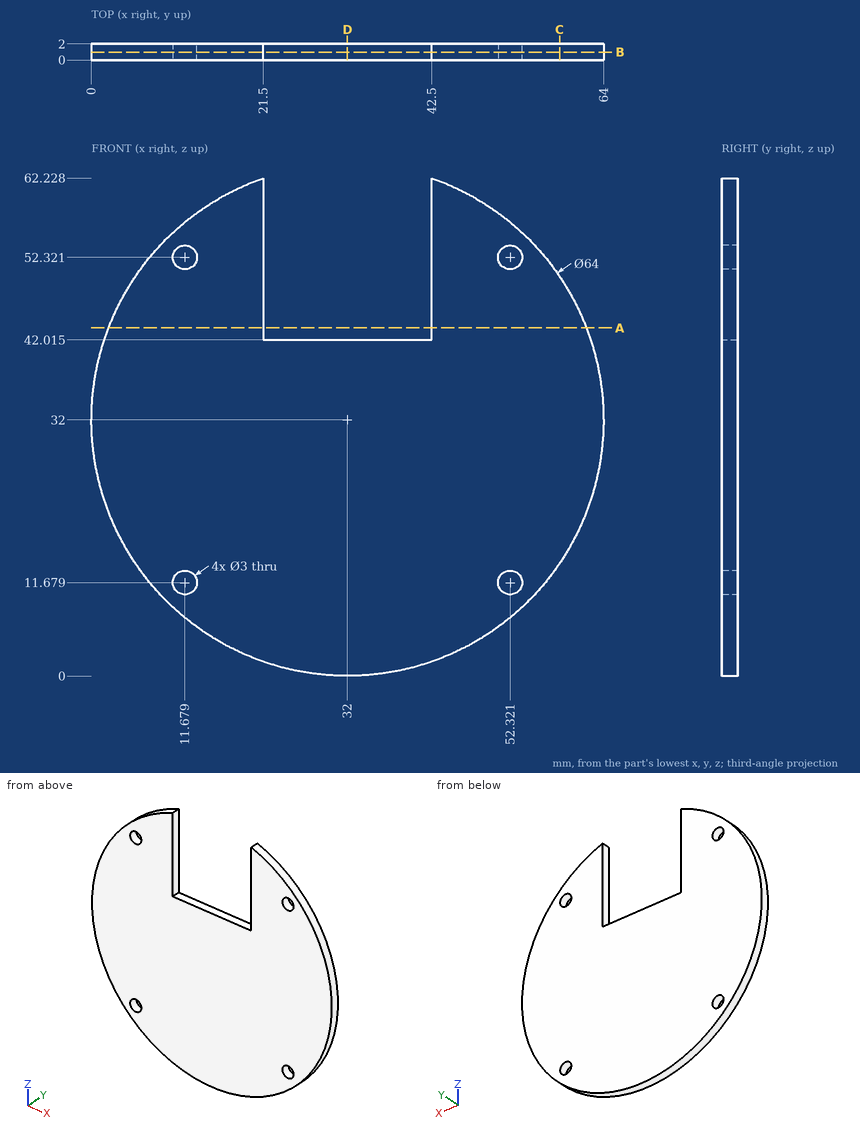
Here's the drawing with two shaded views (mm, measured from the low corner). I have some questions. Coordinates: 2 decimals unless noted, no trailing zeros. Order: outer loops, then holes, each group sorted by start corner. A loop starts at its lowest first (then second) coordinate and runs counter-clockwise, first axis right, second up. Notation, with made-up numbers: (2, 40.5) -> (18, 40.5) arc R27 ccw to (18, 56.5) -> close; hole circle Ø4 at (6, 18). An arc over 180 degrees is marked (long way). One line per question, with ' | ' between items.
Q1. Imagine slicing it at B-B on y = 1. Please give me the cut outline in (x, z) (1 decimal), and give its area (3 significant figures).
Return value:
outline: (21.5, 42) -> (21.5, 62.2) arc R32 ccw (long way) to (42.5, 62.2) -> (42.5, 42) -> close; hole circle Ø3 at (11.7, 11.7); hole circle Ø3 at (11.7, 52.3); hole circle Ø3 at (52.3, 11.7); hole circle Ø3 at (52.3, 52.3) | area: 2,740 mm²
Q2. If I drill on L1, parallel to X at y = 1.6, z = 52 (1 decimal); L2, parallel to Z at x = 51.5, y = 0.3 (1 decimal); L3, parallel to X at y = 1.1, z = 56 (1 decimal), over which ranges is the centre line in solid material (lowest first)?
Return value:
L1: 7 to 10.2, 13.1 to 21.5, 42.5 to 50.9, 53.8 to 57 | L2: 6.6 to 10.4, 12.9 to 51.1, 53.6 to 57.4 | L3: 10.8 to 21.5, 42.5 to 53.2
Q3. Imagine slicing it at A-A on z = 43.5. Please give me the cut outline in (x, y).
Return value:
outline: (2.14, 0) -> (21.5, 0) -> (21.5, 2) -> (2.14, 2) -> close; (42.5, 0) -> (61.86, 0) -> (61.86, 2) -> (42.5, 2) -> close
Q4. I'm going to push flat-ended pins straight in: P1, Ø3.5, axis at x = 11.68, z = 52.32, coming from the -Y side; P2, Ø1, axis at y = 1, z = 57, coming from the -X side (1 decimal); P3, Ø0.6, axis at y = 0.5, z = 52, coming from the +X side; P4, Ø0.6, axis at x = 31, y = 1.5, coming from the +Z side (1 decimal). Where does each tip first touch, or does it pass through?
Return value:
P1: y = 0 | P2: x = 11.4 | P3: x = 57.22 | P4: z = 42
Q5. Imagine slicing it at D-D on x = 32. Please give me the cut outline in (y, z) (1 decimal).
Return value:
outline: (0, 0) -> (2, 0) -> (2, 42) -> (0, 42) -> close
Q6. Imagine slicing it at C-C on x = 58.5. Please give me the cut outline in (y, z).
Return value:
outline: (0, 14.06) -> (2, 14.06) -> (2, 49.94) -> (0, 49.94) -> close
